Input: part model. Units: mm. Frame: model coordinates. A direction names the side the tool comes from. Give positions to 0.01 mm unless a question says otherwise; leave off trailing zeros. Loops run counter-clockwise (first coordinate to the right, second up) from the corner with the lowest first, then second, coordinate; pieces in that order, holes last. Notation, with made-up numbers: M -36,-19 L 9,-19 A21 ccw 9,0 Z; hole C -39.75,28.25 d4. An arc over 180 degrees is marked long. One line per item, written item: value. Start each with the question number.
(1) Section A-A on z = 88.9. Output: boundary loops of the cut face in (x, y), plus the area to 3 significant figures.
(2) Access query for faces 5 (the cylindrical face through (3.414, 93.232, 94.254)), 6 (the cylindrical face through (-1.38, 6.2, -12.52)), 7 (the cylindrical face through (-93.232, 3.414, 94.254)). Directions: +Z, -Z, +X, -X, +Y, -Y. A direction counts if a zero-diameter tool reaches every point of the face in a straight line with its end or side. Return the directions, or none.
(3) Ray query, line 1 along Z through (x, y) = (0.5, 95.5); line 2 along Y through (x, z) = (-49.5, 38); line 3 along Z through (x, y) = (-43, 1.5). Return the intervals inside material, ascending. Write a range as from..to.
(4) Pull-direction query (Z, two-part tool) for faces 1 (the cylindrical face through (95.567, 3.414, 94.254)), 2 (the cylindrical face through (3.414, -95.567, 94.254)), 3 (the flat face through (3, 6, 0)), 4 (the flat face through (0, 177.8, 38)); classes: released by +Z, released by -Z, zero draft, split by the parting line, or undercut.
(5) Section D-D on y = -118. Output: boundary loops of the cut face in (x, z).
(6) Pin query (flat end, axial travel): P1, Ø5, axis at y = 79.5, z = 94.5, coming from the +X side; P2, Ø10, axis at y = -14, z = 78, coming from the -X side. Return the tip coordinate at first contact, or that it passes through.
(7) Section B-B on y = 0. Output: boundary loops of the cut face in (x, z).
```python
from build123d import *

# Parameters (mm, degrees)
F0_R     = 12.7
F1_DEPTH = 152.4
F2_R     = 6.35
F3_DEPTH = 25.4
F5_R     = 6.35
F4_R     = 6.35
F6_DEPTH = 177.8
F7_R     = 6.35
F8_DEPTH = 177.8


with BuildPart() as f1:
    # F0 (on Top) → F1 (new body)
    with BuildSketch(Plane.XY):
        Circle(F0_R)
    extrude(amount=F1_DEPTH)

    # F2 (on face) → F3 (join)
    with BuildSketch(Plane(origin=(0, 0, 0), x_dir=(1, 0, 0), z_dir=(0, 0, -1))):
        Circle(F2_R)
    extrude(amount=F3_DEPTH)

    # F5 (on Front) + F4 (on Front) → F6 (join, symmetric)
    with BuildSketch(Plane.XZ):
        with Locations((0, 38.1)):
            Circle(F5_R)
    with BuildSketch(Plane.XZ):
        with Locations((0, 88.9)):
            Circle(F4_R)
    extrude(amount=F6_DEPTH, both=True)

    # F7 (on Right) → F8 (join, symmetric)
    with BuildSketch(Plane.YZ):
        with Locations((0, 38.1)):
            Circle(F7_R)
        with Locations((0, 88.9)):
            Circle(F7_R)
    extrude(amount=F8_DEPTH, both=True)


solid = f1.part
```
Output values:
1. outline: M -177.8,-6.35 L -11,-6.35 A12.7 ccw -6.35,-11 L -6.35,-177.8 L 6.35,-177.8 L 6.35,-11 A12.7 ccw 11,-6.35 L 177.8,-6.35 L 177.8,6.35 L 11,6.35 A12.7 ccw 6.35,11 L 6.35,177.8 L -6.35,177.8 L -6.35,11 A12.7 ccw -11,6.35 L -177.8,6.35 Z
1. area: 8,920 mm²
2. face 5: +Y
2. face 6: -Z
2. face 7: -X
3. line 1: z = 31.77..44.43, 82.57..95.23
3. line 2: y = -6.35..6.35
3. line 3: z = 31.93..44.27, 82.73..95.07
4. face 1: undercut
4. face 2: undercut
4. face 3: released by -Z
4. face 4: zero draft
5. outline: C 0,38.1 d12.7; C 0,88.9 d12.7
6. P1: stops at x = 5.54
6. P2: stops at x = -8.96
7. outline: M -177.8,31.75 L -12.7,31.75 L -12.7,0 L -6.35,0 L -6.35,-25.4 L 6.35,-25.4 L 6.35,0 L 12.7,0 L 12.7,31.75 L 177.8,31.75 L 177.8,44.45 L 12.7,44.45 L 12.7,82.55 L 177.8,82.55 L 177.8,95.25 L 12.7,95.25 L 12.7,152.4 L -12.7,152.4 L -12.7,95.25 L -177.8,95.25 L -177.8,82.55 L -12.7,82.55 L -12.7,44.45 L -177.8,44.45 Z
